from build123d import *

# Parameters (mm, degrees)
SKETCH_W        = 168
SKETCH_H        = 133.4
PAD_DEPTH       = 1.6
SKETCH001_W     = 163.5
SKETCH001_H     = 95
PAD001_DEPTH    = 0.01
POCKET_DEPTH    = 1.601
POCKET001_DEPTH = 1.601
BODY_ROLL_ANGLE = 5


with BuildPart() as part:
    # Sketch → Pad (new body)
    with BuildSketch(Plane.XY):
        Rectangle(SKETCH_W, SKETCH_H)
    extrude(amount=PAD_DEPTH)

    # Sketch001 (on Face6 of Pad) → Pad001 (join)
    with BuildSketch(Plane.XY.offset(1.6)):
        with Locations((0, -13.2)):
            Rectangle(SKETCH001_W, SKETCH001_H)
    extrude(amount=PAD001_DEPTH)

    # Sketch002 (on Face5 of Pad001) → Pocket (cut, through all)
    with BuildSketch(Plane.XY.offset(1.6)):
        with BuildLine():
            ThreePointArc((-76.5, -61.965896), (-78.1, -63.565896), (-76.5, -65.165896))
            Line((-76.5, -65.165896), (-72.75134, -65.165896))
            ThreePointArc((-72.75134, -65.165896), (-71.15134, -63.565896), (-72.75134, -61.965896))
            Line((-76.5, -61.965896), (-72.75134, -61.965896))
        make_face()
    extrude(amount=-POCKET_DEPTH, mode=Mode.SUBTRACT)

    # Sketch003 (on Face5 of Pocket) → Pocket001 (cut, through all)
    with BuildSketch(Plane.XY.offset(1.6)):
        with BuildLine():
            ThreePointArc((73.5, -62.1), (71.9, -63.7), (73.5, -65.3))
            Line((73.5, -65.3), (76.5, -65.3))
            ThreePointArc((76.5, -65.3), (78.1, -63.7), (76.5, -62.1))
            Line((73.5, -62.1), (76.5, -62.1))
        make_face()
        with BuildLine():
            ThreePointArc((73.5, 65.3), (71.9, 63.7), (73.5, 62.1))
            Line((73.5, 62.1), (76.5, 62.1))
            ThreePointArc((76.5, 62.1), (78.1, 63.7), (76.5, 65.3))
            Line((73.5, 65.3), (76.5, 65.3))
        make_face()
        with BuildLine():
            ThreePointArc((-76.5, 65.3), (-78.1, 63.7), (-76.5, 62.1))
            Line((-76.5, 62.1), (-73.5, 62.1))
            ThreePointArc((-73.5, 62.1), (-71.9, 63.7), (-73.5, 65.3))
            Line((-76.5, 65.3), (-73.5, 65.3))
        make_face()
    extrude(amount=-POCKET001_DEPTH, mode=Mode.SUBTRACT)


with BuildPart() as part_1:
    # Body roll: moved
    add(part.part.rotate(Axis((0, 0, 0), (1, 0, 0)), BODY_ROLL_ANGLE))


with BuildPart() as part_2:
    # Body placement: moved
    add(part_1.part.moved(Location((0, 47.65, 18.82))))


solid = part_2.part
The listing builds one solid part. Answer for the finished solid, in the listing's coordinates (mm). Round coordinates to 2 decimals unless told otherwise and drop trailing zeros. Write each loop counter-clockwise with the first axis right and the second up, starting at its lowest first coordinate (ties: lowest second). Pieces come first, ordered by that corner, then holes. Notation, with made-up numbers: (-21, 25) - (11, 25) arc R14 cw to (11, 48) - close; hole circle Ø4 at (7.25, -28). An arc over 180 degrees is marked (long way). Use a Markdown table: item, result. Add a question column.
1. Flat-ended cylindrical pins translate along their axes: P1, Ø12, axis at x = -34.5, y = 54.5, coming from the -Z side; P2, Ø1, axis at x = -39, y = 41.5, coming from the +Z side. Find the tip coordinate at first contact, or state that the pin passes through.
2. The part is cut by section C-C (y = 94). Write down the section's boundary in (x, z), and give its area (3 significant figures).
3. Consider line 1 (Z direction, x = 48.5, y = 4); line 2 (Z direction, x = 0, y = -12.5). Determine where each line is inside the solid, lowest interval first.
Reported:
| question | item | result |
|---|---|---|
| 1 | P1 | z = 18.89 |
| 1 | P2 | z = 19.94 |
| 2 | outline | (-84, 22.88) - (84, 22.88) - (84, 24.48) - (-84, 24.48) - close |
| 2 | area | 270 mm^2 |
| 3 | line 1 | 15 to 16.62 |
| 3 | line 2 | 13.56 to 15.17 |
